Source: CAD feature listing. Evaluate the final solid. Frame: model axes, mm. A direction names the side the tool comes from. Round coordinates to 2 decimals unless told otherwise and drop trailing zeros. Loops run counter-clockwise (first coordinate to the right, second up) from the corner with the lowest first, then second, coordinate; pieces in that order, holes last. Notation, with made-up numbers: (22, 13) -> (45, 13) arc R25 cw to (45, 50) -> close; hole circle Ø6 at (0, 14). An arc over 180 degrees is marked (long way). Return JSON: item names as keys, results as strings. Group by question number.
Solid Edge part; units mm, degrees
sketch "Sketch1" plane through (0, 0, 0) normal (0, -1, 0) x (1, 0, 0)
  circle A0 centre (0, 0) radius 16
extrude "ExtrudedProtrusion_1" add sketch "Sketch1" along normal mid plane 56
sketch "Sketch2" plane through (0, 0, 0) normal (0, 0, 1) x (1, 0, 0)
  circle A0 centre (18, 0) radius 16
extrude "ExtrudedProtrusion_2" add sketch "Sketch2" along normal mid plane 56
sketch "Sketch3" plane through (0, 28, 0) normal (0, 1, 0) x (1, 0, 0)
  circle A0 centre (0, 0) radius 8
extrude "ExtrudedCutout_1" cut sketch "Sketch3" along normal mid plane 203.9389
sketch "Sketch4" plane through (18, 0, 28) normal (0, 0, 1) x (0, 1, 0)
  circle A0 centre (0, 0) radius 8
extrude "ExtrudedCutout_2" cut sketch "Sketch4" along normal mid plane 249.3799
fillet "Round_1" radius 2 1 edges at (9, -13.2288, 13.2288)
(1) Mould query, pull axis X, two halves, no side actions, for faces 3 (the face through (14.2, 7.3, -28)), 4 (the face through (-1.73, 0.39, 7.81)). Classes: released by +X, released by -X, zero draft, split by the parting line, or undercut.
(2) Cut plane A-A (y = 0). Count the separate pieces of the cut face and the enclosed holes in it, and give its area (3 significant figures).
(3) Cut plane D-D (x = 30). Return loops of the section in (y, z), and give its area (3 significant figures).
(4) Set-up query: faces 1 (the face through (-15.985, 0.392, -0.703)), 2 (the face through (14.2, 7.3, 28)). Return all of +Z, -Z, +X, -X, +Y, -Y with unobstructed straight access to the full face (end or side cutting, diameter ignored); none if empty.
(5) Ray query, line 1 (Y direction, x = 18, z = 16); line 2 (Y direction, x = 14, z = 24). Return the intervals inside material, ascending.
(6) Cut plane C-C (y = 24.5). Return loops of the section in (x, z).
(7) Pin query (flat end, axial travel): pin 1 (2 mm diameter, centred on y = -19, z = 10, fed in from +X); pin 2 (2 mm diameter, centred on x = 14.5, z = -16, fed in from +Y); pin 3 (3 mm diameter, centred on y = -13.5, z = -5.5, fed in from +X); pin 4 (9.5 mm diameter, centred on x = 18, y = 0, fed in from +Z). Return the tip coordinate at first contact, or that it passes through.
Answers follow:
{
 "1": {"face 3": "zero draft", "face 4": "undercut"},
 "2": {"separate pieces": "2", "enclosed holes": "1", "area": "1,160 mm^2"},
 "3": {"outline": "(-10.58, -28) -> (10.58, -28) -> (10.58, 28) -> (-10.58, 28) -> close", "area": "1,190 mm^2"},
 "4": {"face 1": "none", "face 2": "+Z, +X, -X, +Y, -Y"},
 "5": {"line 1": "-16 to -8, 8 to 16", "line 2": "-15.49 to -6.93, 6.93 to 15.49"},
 "6": {"outline": "circle Ø32 at (0, 0); hole circle Ø16 at (0, 0)"},
 "7": {"pin 1": "x = 13.23", "pin 2": "y = 15.8", "pin 3": "x = 28.58", "pin 4": "through"}
}
